Verification items for the finished model (mm, model axes). Round coordinates to 2 decimals unless told otherwise and drop trailing zeros. Write each loop counter-clockwise with the first axis right and the second up, starting at its lowest first coordinate (ties: lowest second). Pieces come first, ordered by that corner, then holes. Notation, with made-up numbers: (14, 80) -> (58, 80) arc R33 ccw to (58, 116) -> close; hole circle Ø7 at (65.25, 88.25). An arc over 180 degrees is marked (long way). Answer as a JSON object with one key per item and string values. Group by question number.
(1) Sectioned sample at A-A on y = 1.1. Count the separate pieces of the cut face and the enclosed holes in it, and give its area (3 significant figures).
(2) Gauge pin test, flat end, axial feed: pin 1 Ø4 at (x, z) = (-93, -40) entering from -Y. Record the tip position at first contact, or that the pin passes through.
(3) Sectioned sample at B-B on x = -63.5. Record the cut outline in (y, z), and give its area (3 significant figures).
(4) Scan lines: L1, parallel to X at y = 1.6, z = -40; L2, parallel to X at y = 3.7, z = 88; L3, parallel to X at y = 3.05, z = 34. Record each from-to range of solid material in increasing order. Write a range as from..to.
```python
from build123d import *

# Parameters (mm, degrees)
BOSS_EXTRUDE1_DEPTH = 4
SKETCH2_R           = 2.5
SKETCH2_R_2         = 2.1
CUT_EXTRUDE1_DEPTH  = 227.373585031
SKETCH3_W           = 15
SKETCH3_H           = 35
CUT_EXTRUDE2_DEPTH  = 227.373585031
SKETCH4_R           = 2.1
CUT_EXTRUDE3_DEPTH  = 10
CHAMFER1_SIZE       = 20
FILLET1_R           = 5


with BuildPart() as part:
    # Sketch1 → Boss-Extrude1 (new body)
    with BuildSketch(Plane(origin=(0, 0, 0), x_dir=(1, 0, 0), z_dir=(0, 1, 0))):
        Polygon((-123, 125), (8, 125), (8, 190), (53, 190), (53, 125), (53, -125), (-53, -125), (-123, -125), align=None)
    extrude(amount=BOSS_EXTRUDE1_DEPTH)

    # Sketch2 → Cut-Extrude1 (cut, through all)
    with BuildSketch(Plane(origin=(0, 4, 0), x_dir=(1, 0, 0), z_dir=(0, 1, 0))):
        with Locations(Location((-110.5, -112.5, 0), (0, 0, 270))):
            Circle(SKETCH2_R)
        with Locations(Location((-75.5, -112.5, 0), (0, 0, 270))):
            Circle(SKETCH2_R)
        with Locations(Location((-93, -112.5, 0), (0, 0, 270))):
            Circle(SKETCH2_R)
        with Locations(Location((-93, -87.5, 0), (0, 0, 270))):
            Circle(SKETCH2_R_2)
        with Locations(Location((5.5, -112.5, 0), (0, 0, 270))):
            Circle(SKETCH2_R)
        with Locations(Location((23, -112.5, 0), (0, 0, 270))):
            Circle(SKETCH2_R)
        with Locations(Location((40.5, -112.5, 0), (0, 0, 270))):
            Circle(SKETCH2_R)
        with Locations(Location((23, -87.5, 0), (0, 0, 270))):
            Circle(SKETCH2_R_2)
        with Locations(Location((23, 87.5, 0), (0, 0, 90))):
            Circle(SKETCH2_R_2)
        with Locations(Location((40.5, 112.5, 0), (0, 0, 90))):
            Circle(SKETCH2_R)
        with Locations(Location((23, 112.5, 0), (0, 0, 90))):
            Circle(SKETCH2_R)
        with Locations(Location((5.5, 112.5, 0), (0, 0, 90))):
            Circle(SKETCH2_R)
        with Locations(Location((-93, 87.5, 0), (0, 0, 90))):
            Circle(SKETCH2_R_2)
        with Locations(Location((-93, 112.5, 0), (0, 0, 90))):
            Circle(SKETCH2_R)
        with Locations(Location((-75.5, 112.5, 0), (0, 0, 90))):
            Circle(SKETCH2_R)
        with Locations(Location((-110.5, 112.5, 0), (0, 0, 90))):
            Circle(SKETCH2_R)
        with Locations(Location((40.5, 172.5, 0), (0, 0, 270))):
            Circle(SKETCH2_R)
        with Locations(Location((23, 172.5, 0), (0, 0, 270))):
            Circle(SKETCH2_R)
    extrude(amount=-CUT_EXTRUDE1_DEPTH, mode=Mode.SUBTRACT)

    # Sketch3 → Cut-Extrude2 (cut, through all)
    with BuildSketch(Plane.XZ):
        with Locations((-34.5, 37.5)):
            Rectangle(SKETCH3_W, SKETCH3_H)
        with Locations((-34.5, -37.5)):
            Rectangle(SKETCH3_W, SKETCH3_H)
    extrude(amount=-CUT_EXTRUDE2_DEPTH, mode=Mode.SUBTRACT)

    # Sketch4 → Cut-Extrude3 (cut)
    with BuildSketch(Plane.XZ):
        with Locations(Location((-93, 40, 0), (0, 0, 270))):
            Circle(SKETCH4_R)
        with Locations(Location((-93, -40, 0), (0, 0, 90))):
            Circle(SKETCH4_R)
        with Locations(Location((23, -40, 0), (0, 0, 270))):
            Circle(SKETCH4_R)
        with Locations(Location((23, 40, 0), (0, 0, 90))):
            Circle(SKETCH4_R)
    extrude(amount=-CUT_EXTRUDE3_DEPTH, mode=Mode.SUBTRACT)

    # Chamfer1
    chamfer1_edges = [part.edges().sort_by_distance(p)[0] for p in [
        (8, 2, -125),
    ]]
    chamfer(chamfer1_edges, length=CHAMFER1_SIZE)

    # Fillet1
    fillet1_edges = [part.edges().sort_by_distance(p)[0] for p in [
        (-123, 2, -125),
        (8, 2, -190),
        (53, 2, -190),
        (53, 2, 125),
        (-123, 2, 125),
        (-12, 2, -125),
        (8, 2, -145),
    ]]
    fillet(fillet1_edges, radius=FILLET1_R)


solid = part.part
```
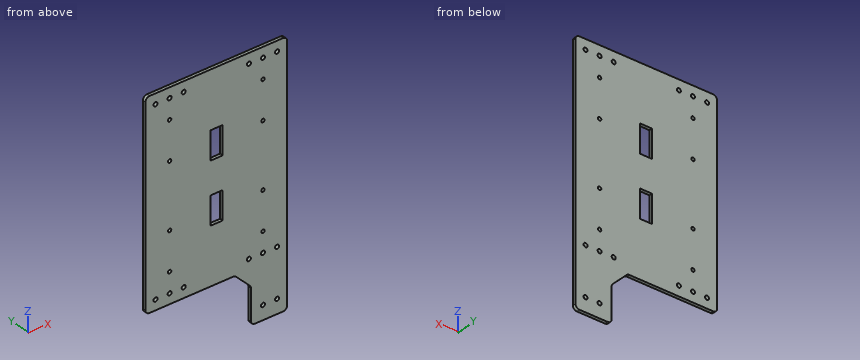
Computed values:
{
 "1": {"separate pieces": "1", "enclosed holes": "24", "area": "45,700 mm2"},
 "2": {"pin 1": "through"},
 "3": {"outline": "(0, -125) -> (4, -125) -> (4, 125) -> (0, 125) -> close", "area": "1,000 mm2"},
 "4": {"L1": "-123..-95.1, -90.9..-42, -27..20.9, 25.1..53", "L2": "-123..-95.04, -90.96..20.96, 25.04..53", "L3": "-123..-42, -27..53"}
}
